Geometry: final body of the model. Coordinates: model frame, mm. Face numbers are marked on the shaded views. Round coordinates to 2 decimals unless told otherwise and drop trailing zeros. Loops run counter-clockwise (first coordinate to the right, second up) from the corner with the lowest first, then second, coordinate; pieces in that order, holes last. Notation, with made-up numbers: (52, 39.25) -> (108, 39.25) arc R13 ccw to (108, 45.25) -> close; hole circle Ø2 at (80, 85). An arc over 180 degrees is marked (long way). Answer in a Markdown table with one row per item.
```python
from build123d import *

# Parameters (mm, degrees)
SKETCH1_W           = 33.895402138
SKETCH1_H           = 12
SKETCH1_R           = 3
BOSS_EXTRUDE1_DEPTH = 10
FILLET1_R           = 6


with BuildPart() as part:
    # Sketch1 → Boss-Extrude1 (new body)
    with BuildSketch(Plane(origin=(0, 0, 0), x_dir=(1, 0, 0), z_dir=(0, 1, 0))):
        with Locations((16.947701069, 0)):
            Rectangle(SKETCH1_W, SKETCH1_H)
        with Locations(Location((28.9, 0, 0), (0, 0, 270))):
            Circle(SKETCH1_R, mode=Mode.SUBTRACT)
    extrude(amount=BOSS_EXTRUDE1_DEPTH)

    # Fillet1
    fillet1_edges = [part.edges().sort_by_distance(p)[0] for p in [
        (33.895402138, 5, -6),
        (33.895402138, 5, 6),
    ]]
    fillet(fillet1_edges, radius=FILLET1_R - 0.0001)  # a hair under: the kernel refuses the full size


solid = part.part
```
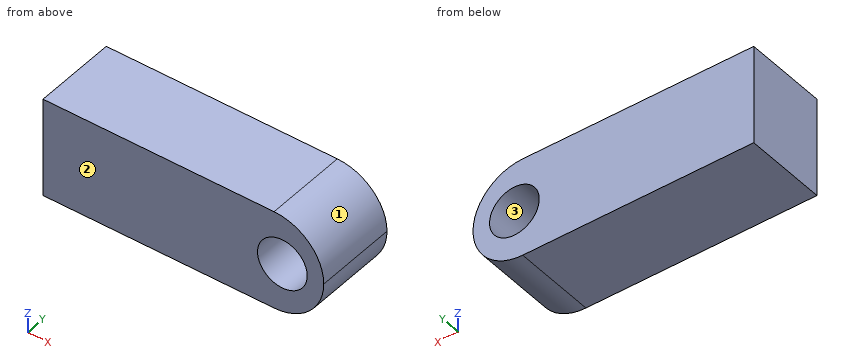
Item 1: Ray query, L1, parallel to X at y = 5.5, z = 0; L2, parallel to X at y = 3.75, z = -1; L3, parallel to X at y = 8.25, z = -3.25. Return the intervals inside material, ascending.
Ans:
| item | result |
|---|---|
| L1 | 0 to 25.9, 31.9 to 33.9 |
| L2 | 0 to 26.07, 31.73 to 33.81 |
| L3 | 0 to 32.94 |
Item 2: Mould query, pull axis Z, two halves, no side actions, for the marked faces 1, 2 and 3. Classes: released by +Z, released by -Z, zero draft, split by the parting line, or undercut.
Ans:
| item | result |
|---|---|
| face 1 | released by +Z |
| face 2 | zero draft |
| face 3 | undercut |
Item 3: Section query C-C, the plane z = -2.5. Output: boundary loops of the cut face in (x, y), and give its area (3 significant figures).
Ans:
| item | result |
|---|---|
| outline | (0, 0) -> (27.24, 0) -> (27.24, 10) -> (0, 10) -> close; (30.56, 0) -> (33.35, 0) -> (33.35, 10) -> (30.56, 10) -> close |
| area | 300 mm2 |
Item 4: Section query A-A, the plane x = 28.9. Output: boundary loops of the cut face in (y, z), and give its area (3 significant figures).
Ans:
| item | result |
|---|---|
| outline | (0, -5.92) -> (10, -5.92) -> (10, -3) -> (0, -3) -> close; (0, 3) -> (10, 3) -> (10, 5.92) -> (0, 5.92) -> close |
| area | 58.3 mm2 |
Item 5: Section query D-D, the plane z = 4.5. Output: boundary loops of the cut face in (x, y).
Ans:
| item | result |
|---|---|
| outline | (0, 0) -> (31.86, 0) -> (31.86, 10) -> (0, 10) -> close |
Item 6: First-contact query: P1, Ø1.5, axis at y = 9, z = 4, coming from the +X side; P2, Ø3, axis at x = 29, y = 5.5, coming from the -Z side; P3, Ø4, axis at y = 1.5, z = -2.5, coming from the +X side. Flat tips, straight axial feed; report the tip coordinate or a pass-through.
Ans:
| item | result |
|---|---|
| P1 | x = 32.94 |
| P2 | z = -6 |
| P3 | x = 33.87 |
